```python
from build123d import *

# Parameters (mm, degrees)
SKETCH_1_R               = 15
EXTRUDE_1_DEPTH          = 3
CUT_EXTRUDE_2_DEPTH      = 22.424285286
CUT_EXTRUDE_2_DEPTH_BACK = 22.424285286
SKETCH_3_R               = 1.5
CUT_EXTRUDE_3_DEPTH      = 3
SKETCH_4_R               = 0.5
CUT_EXTRUDE_4_DEPTH      = 3


with BuildPart() as part:
    # 草图1 → 凸台-拉伸1 (new body)
    with BuildSketch(Plane(origin=(0, 0, 0), x_dir=(1, 0, 0), z_dir=(0, 1, 0))):
        with Locations(Location((0, 0, 0), (0, 0, 270))):
            Circle(SKETCH_1_R)
    extrude(amount=EXTRUDE_1_DEPTH)

    # 草图2 → 切除-拉伸2 (cut, two sides: drawn at the far end of the back side and taken through both)
    with BuildSketch(Plane.XY.offset(-CUT_EXTRUDE_2_DEPTH_BACK)):
        Polygon((-6, 55.426406871), (-6, 3), (-6, 2), (6, 2), (6, 3), (6, 55.426406871), (6, 160.279220614), (-6, 160.279220614), align=None)
    extrude(amount=CUT_EXTRUDE_2_DEPTH + CUT_EXTRUDE_2_DEPTH_BACK, mode=Mode.SUBTRACT)

    # 草图3 → 切除-拉伸3 (cut)
    with BuildSketch(Plane(origin=(0, 3, 0), x_dir=(1, 0, 0), z_dir=(0, 1, 0))):
        with Locations(Location((12.5, 0, 0), (0, 0, 270))):
            Circle(SKETCH_3_R)
        with Locations(Location((-12.5, 0, 0), (0, 0, 90))):
            Circle(SKETCH_3_R)
    extrude(amount=-CUT_EXTRUDE_3_DEPTH, mode=Mode.SUBTRACT)

    # 草图4 → 切除-拉伸4 (cut)
    with BuildSketch(Plane(origin=(0, 3, 0), x_dir=(1, 0, 0), z_dir=(0, 1, 0))):
        with Locations(Location((8.485281374, 8.485281374, 0), (0, 0, 270))):
            Circle(SKETCH_4_R)
        with Locations(Location((-8.485281374, 8.485281374, 0), (0, 0, 90))):
            Circle(SKETCH_4_R)
        with Locations(Location((8.485281374, -8.485281374, 0), (0, 0, 90))):
            Circle(SKETCH_4_R)
        with Locations(Location((-8.485281374, -8.485281374, 0), (0, 0, 270))):
            Circle(SKETCH_4_R)
    extrude(amount=-CUT_EXTRUDE_4_DEPTH, mode=Mode.SUBTRACT)


solid = part.part
```
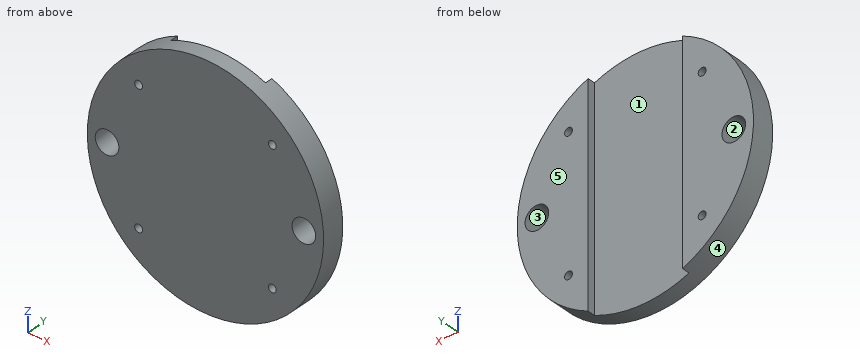
Design review of the part built by this model. Coordinates are the model's own, in mm. Face numbers are marked on the shaded views. A direction names the side the tool comes from. Coordinates: 2 decimals unless noted, no trailing zeros. Order: outer loops, then holes, each group sorted by start corner. A loop starts at its lowest first (then second) coordinate and runs counter-clockwise, first axis right, second up.
1) For the marked faces 1 and 2, list the 3-axis set-ups (+Z, -Z, +X, -X, +Y, -Y) from which the entire face can be reached by the end or side of a thin tool; tool diameter is ignored.
2) Take a section at B-B, the plane x = -12.5. Give the boundary of the cut face in (y, z), and give its area (3 significant figures).
3) Mouldability with a two-part tool opening along X and no side actions: class the marked faces 3, 4 and 5 as +X half, -X half, draft (parallel to the pull), parting line (faces both ways), or undercut.
4) Wall thickness on line 1 along X through (y, z) = (1.15, 0); line 2 along Y through (x, z) = (5, 0.25); line 3 along X through (y, z) = (2.55, 6): over which ranges is each line inside the solid? List them lowest first.
5) Clearance check with flat-ended pins moving along their axes: pin 1 (5 mm diameter, centred on x = 0.5, z = -11.5, fed in from -Y); pin 2 (1 mm diameter, centred on y = 0.5, z = -5, fed in from +X); pin 3 (1.8 mm diameter, centred on x = -12.5, z = 0, fed in from +Y); pin 4 (0.5 mm diameter, centred on y = 2.5, z = -1, fed in from +X). State where each tip first meets the part, or that it passes through.
6) Take a section at C-C, the plane y = 0.75. Give the boundary of the cut face in (x, z).
7) Take a section at A-A, the plane z = 0. Give the boundary of the cut face in (x, y).
8) Take a section at D-D, the plane z = 10. Give the boundary of the cut face in (x, y).
Returned:
1. face 1: +Z, -Z, +Y
1. face 2: +Y, -Y
2. outline: (0, -8.29) - (3, -8.29) - (3, -1.5) - (0, -1.5) - close; (0, 1.5) - (3, 1.5) - (3, 8.29) - (0, 8.29) - close
2. area: 40.7 mm2
3. face 3: undercut
3. face 4: parting line
3. face 5: draft
4. line 1: x = -15 to -14, -11 to 11, 14 to 15
4. line 2: y = 0 to 2
4. line 3: x = -13.75 to -6, 6 to 13.75
5. pin 1: stops at y = 0
5. pin 2: stops at x = 14.31
5. pin 3: passes through
5. pin 4: stops at x = 14.98
6. outline: circle Ø30 at (0, 0); hole circle Ø3 at (-12.5, 0); hole circle Ø1 at (-8.49, -8.49); hole circle Ø1 at (-8.49, 8.49); hole circle Ø1 at (8.49, -8.49); hole circle Ø1 at (8.49, 8.49); hole circle Ø3 at (12.5, 0)
7. outline: (-15, 0) - (-14, 0) - (-14, 3) - (-15, 3) - close; (-11, 0) - (11, 0) - (11, 3) - (6, 3) - (6, 2) - (-6, 2) - (-6, 3) - (-11, 3) - close; (14, 0) - (15, 0) - (15, 3) - (14, 3) - close
8. outline: (-11.18, 0) - (11.18, 0) - (11.18, 3) - (6, 3) - (6, 2) - (-6, 2) - (-6, 3) - (-11.18, 3) - close
